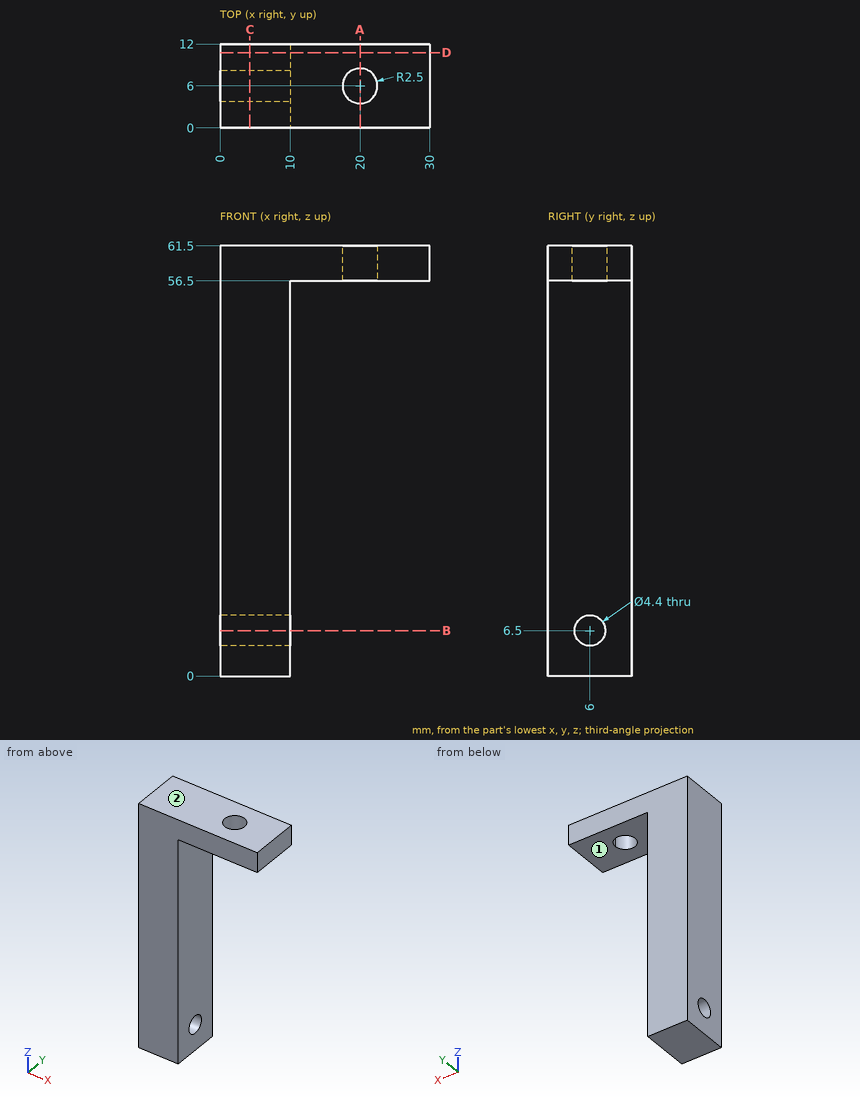
The drawing under review shows one solid part. Ordinate dimensions are in mm from its lowest x, y, z. A direction names the side the tool comes from. Give positions to 0.01 mm unless a question says otherwise; leave off trailing zeros. Order: outer loops, then holes, each group sorted by start corner. A loop starts at its lowest first (then second) coordinate and runs counter-clockwise, first axis right, second up. Notation, with made-up numbers: M -32.5,17 L -26.5,17 A31 ccw -26.5,50 Z; hole C 30.5,-22.75 d2. An arc over 180 degrees is marked long. Answer in a Markdown table with one row per item. Add a question column.
1. Add section B-B on z = 6.5. State the section outline as (x, y) points, plus the area to 3 significant figures.
2. For pin 1 Ø3 at (y, z) = (8.5, 23.5) entering from +X; pin 2 Ø5 at (x, y) = (25, 10) entering from -Z; pin 3 Ø4 at (y, z) = (6, 6.5) entering from -X, all flat-tipped, find the tip position at first contact; note any pin that passes through.
3. To check wall thickness, follow line 1 along Z through (x, y) = (7.75, 6); line 2 along Z through (x, y) = (17.5, 0.5); line 3 along X through (y, z) = (8.75, 23). State the ranges of each line that lie inside material, in increasing order.
4. Machinability: for the marked faces 1 and 2, which of the approach directions +Z, -Z, +X, -X, +Y, -Y give a long, thin tool a straight path to every point of the face, cutting with its end or side? Answer none if there is none.
5. Add section D-D on y = 10.75. State the section outline as (x, z) points.
6. Add section C-C on x = 4.25. State the section outline as (y, z) points, plus the area to 3 significant figures.
7. Add section A-A on x = 20. State the section outline as (y, z) points.
The answers:
| question | item | result |
|---|---|---|
| 1 | outline | M 0,0 L 10,0 L 10,3.8 L 0,3.8 Z; M 0,8.2 L 10,8.2 L 10,12 L 0,12 Z |
| 1 | area | 76.0 mm2 |
| 2 | pin 1 | x = 10 |
| 2 | pin 2 | z = 56.5 |
| 2 | pin 3 | through |
| 3 | line 1 | 0 to 4.3, 8.7 to 61.5 |
| 3 | line 2 | 56.5 to 61.5 |
| 3 | line 3 | 0 to 10 |
| 4 | face 1 | -Z, +X, +Y, -Y |
| 4 | face 2 | +Z, +X, -X, +Y, -Y |
| 5 | outline | M 0,0 L 10,0 L 10,56.5 L 30,56.5 L 30,61.5 L 0,61.5 Z |
| 6 | outline | M 0,0 L 12,0 L 12,61.5 L 0,61.5 Z; hole C 6,6.5 d4.4 |
| 6 | area | 723 mm2 |
| 7 | outline | M 0,56.5 L 3.5,56.5 L 3.5,61.5 L 0,61.5 Z; M 8.5,56.5 L 12,56.5 L 12,61.5 L 8.5,61.5 Z |
